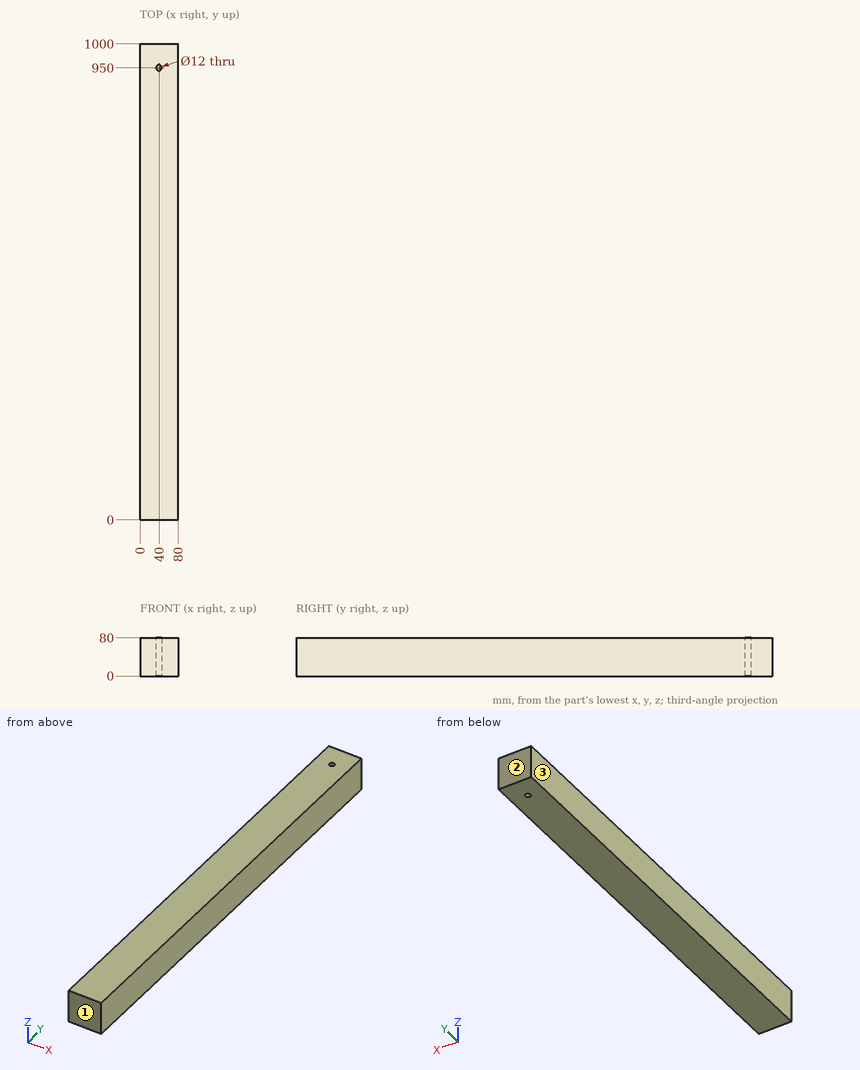
Answer from the drawing. Dimensions are ordinates in mm from the lowest x, y and z of the part. Round coordinates to 2 decimals unless told otherwise and drop trailing zeros. Write each question's results on one line, items separated by ' | '. Start each with the question number.
Item 1: The mould has two halves that part along Y. Classify the marked faces 1, 2 and 3: +Y half, -Y half, draft (parallel to the pull), parting line (faces both ways), or undercut.
Item 2: Straight lines are drawn through the part: probe 1 along Y at (x, z) = (40, 54); probe 2 along X at (y, z) = (950, 44); probe 3 along Y at (x, z) = (38, 72.5). For each, find the intervals that lie inside material, in ascending order.
Item 3: Given pin 1 Ø1 at (y, z) = (590.5, 42.5) entering from -X; pin 2 Ø11 at (x, y) = (40, 950) entering from -Z, each flat-ended and moving along its own axis, determine where each tip first touches the part or whether it passes through.
Answer block:
1) face 1: -Y half | face 2: +Y half | face 3: draft
2) probe 1: y = 0 to 944, 956 to 1000 | probe 2: x = 0 to 34, 46 to 80 | probe 3: y = 0 to 944.34, 955.66 to 1000
3) pin 1: stops at x = 0 | pin 2: passes through
